from build123d import *

# Parameters (mm, degrees)
BOSS_EXTRUDE1_DEPTH = 4.125
SKETCH2_R           = 5
BOSS_EXTRUDE2_DEPTH = 0.5
SKETCH3_R           = 3.5
CUT_EXTRUDE1_DEPTH  = 9
SKETCH4_R           = 0.375
CUT_EXTRUDE2_DEPTH  = 0.5
CIRPATTERN1_COUNT   = 3
BOSS_EXTRUDE3_START = 6.5
BOSS_EXTRUDE3_DEPTH = 6.5
SKETCH7_R           = 3.5
BOSS_EXTRUDE4_DEPTH = 6.5
SKETCH8_R           = 3
CUT_EXTRUDE3_DEPTH  = 9
SKETCH6_R           = 0.75
CUT_EXTRUDE4_DEPTH  = 9


with BuildPart() as part:
    # Sketch1 → Boss-Extrude1 (new, symmetric)
    with BuildSketch(Plane.XY):
        Polygon((3, 0), (-3, 0), (-3, -0.45), (-2.5, -0.45), (-2.5, -0.9), (-3, -0.9), (-3, -1.35), (-2.5, -1.35), (-2.5, -1.8), (-3, -1.8), (-3, -2.25), (-2.5, -2.25), (-2.5, -2.7), (-3, -2.7), (-3, -3.15), (-2.5, -3.15), (-2.5, -3.6), (-3, -3.6), (-3, -4.05), (-2.5, -4.05), (-2.5, -4.5), (-3, -4.5), (-3, -4.95), (-2.5, -4.95), (-2.5, -5.4), (-3, -5.4), (-3, -5.85), (-2.5, -5.85), (-2.5, -6.3), (2.5, -6.3), (2.5, -5.85), (3, -5.85), (3, -5.4), (2.5, -5.4), (2.5, -4.95), (3, -4.95), (3, -4.5), (2.5, -4.5), (2.5, -4.05), (3, -4.05), (3, -3.6), (2.5, -3.6), (2.5, -3.15), (3, -3.15), (3, -2.7), (2.5, -2.7), (2.5, -2.25), (3, -2.25), (3, -1.8), (2.5, -1.8), (2.5, -1.35), (3, -1.35), (3, -0.9), (2.5, -0.9), (2.5, -0.45), (3, -0.45), align=None)
    extrude(amount=BOSS_EXTRUDE1_DEPTH, both=True)

    # Sketch2 → Boss-Extrude2 (add)
    with BuildSketch(Plane.XY.offset(4.125)):
        with Locations(Location((0, -6, 0), (0, 0, 126.869897646))):
            Circle(SKETCH2_R)
    extrude(amount=BOSS_EXTRUDE2_DEPTH)

    # Sketch3 → Cut-Extrude1 (cut)
    with BuildSketch(Plane.XY.offset(4.625)):
        with Locations((0, -6)):
            Circle(SKETCH3_R)
    extrude(amount=-CUT_EXTRUDE1_DEPTH, mode=Mode.SUBTRACT)

    # Sketch4 → Cut-Extrude2 (cut)
    with BuildSketch(Plane.XY.offset(4.625)):
        with Locations((3.464101615, -4)):
            Circle(SKETCH4_R)
    cut_extrude2 = extrude(amount=-CUT_EXTRUDE2_DEPTH, mode=Mode.SUBTRACT)

    # CirPattern1: Cut-Extrude2 ×3 about axis
    cirpattern1_axis = Axis((0, -6, 0), (0, 0, 1))
    for i in range(1, CIRPATTERN1_COUNT):
        add(cut_extrude2.rotate(cirpattern1_axis, i * 360 / CIRPATTERN1_COUNT), mode=Mode.SUBTRACT)

    # Sketch5 → Boss-Extrude3 (add)
    with BuildSketch(Plane.XY.offset(-4.875).offset(BOSS_EXTRUDE3_START)):
        with BuildLine():
            Line((6, -12.75), (-6, -12.75))
            Line((-6, -12.75), (-3.312648335, -4.870238517))
            ThreePointArc((-3.312648335, -4.870238517), (0, -2.5), (3.312648335, -4.870238517))
            Line((3.312648335, -4.870238517), (6, -12.75))
        make_face()
    extrude(amount=-BOSS_EXTRUDE3_DEPTH)

    # Sketch7 → Boss-Extrude4 (add)
    with BuildSketch(Plane.XY.offset(4.625)):
        with Locations(Location((0, -6, 0), (0, 0, 161.168324383))):
            Circle(SKETCH7_R)
    extrude(amount=-BOSS_EXTRUDE4_DEPTH)

    # Sketch8 → Cut-Extrude3 (cut)
    with BuildSketch(Plane.XY.offset(4.625)):
        with Locations((0, -6)):
            Circle(SKETCH8_R)
    extrude(amount=-CUT_EXTRUDE3_DEPTH, mode=Mode.SUBTRACT)

    # Sketch6 → Cut-Extrude4 (cut)
    with BuildSketch(Plane(origin=(0, 0, -4.875), x_dir=(-1, 0, 0), z_dir=(0, 0, -1))):
        with Locations((0, -6)):
            Circle(SKETCH6_R)
    extrude(amount=-CUT_EXTRUDE4_DEPTH, mode=Mode.SUBTRACT)


solid = part.part
Here's how the part is built. I have some questions about the finished solid (model axes, mm). A direction names the side the tool comes from. Round coordinates to 2 decimals unless told otherwise and drop trailing zeros. Order: outer loops, then holes, each group sorted by start corner. A loop starts at its lowest first (then second) coordinate and runs counter-clockwise, first axis right, second up. Notation, with made-up numbers: (-7.5, -37) -> (28.5, -37) arc R13 ccw to (28.5, -30) -> close; hole circle Ø9 at (-27.75, -20). An arc over 180 degrees is marked (long way). Return JSON: item names as keys, results as strings.
Q1. Which directions (+Z, -Z, +X, -X, +Y, -Y) give clear straight access to the entire face, cutting with the end or side of a thin tool? Please do faces 1 (the flat face through (4.638, -8.755, -1.58)), 2 (the flat face through (0, -0.6, 4.125)), 3 (the cylindrical face through (2.82, -10.13, 4.37)), 4 (the flat face through (-2, -3, 4.625)), 5 (the cylindrical face through (0.326, -9.485, 1.979)).
Filled sheet:
{"face 1": "-Z, +X, +Y", "face 2": "+Z, +Y", "face 3": "+Z", "face 4": "+Z, +X, -X, +Y, -Y", "face 5": "none"}
Q2. For pin 1 Ø3.5 at (x, y) = (0, -6) entering from +Z (3 decimals); pin 2 Ø4 at (y, z) = (-3.5, 3) entering from -X; pin 3 Ø4 at (y, z) = (-8, -3) entering from +X, each with a flat end and sliding along its axis, tell me the tip position at first contact or that it passes through.
Filled sheet:
{"pin 1": "stops at z = -4.375", "pin 2": "stops at x = -4.93", "pin 3": "stops at x = 5.06"}
Q3. If we section it at D-D on x = 2: List the corners of the cut face in (y, z) for me (3 decimals).
Filled sheet:
{"outline": "(-12.75, -4.875) -> (-3.128, -4.875) -> (-3.128, -4.125) -> (0, -4.125) -> (0, 4.125) -> (-1.417, 4.125) -> (-1.417, 4.625) -> (-3.764, 4.625) -> (-3.764, -4.375) -> (-8.236, -4.375) -> (-8.236, 4.625) -> (-10.583, 4.625) -> (-10.583, 4.125) -> (-8.872, 4.125) -> (-8.872, 1.625) -> (-12.75, 1.625) -> close"}
Q4. I need wall thicknesses on line 1 along Y through (x, z) = (0, -2.25); line 2 along Z through (x, y) = (0.5, -9.5) (3 decimals); line 3 along Z through (x, y) = (4.75, -5) (3 decimals). Which ranges of each line are inside material? Lowest first, please. Write a range as from..to.
Filled sheet:
{"line 1": "y = -12.75..-9, -3..0", "line 2": "z = -4.875..1.625, 4.125..4.625", "line 3": "z = 4.125..4.625"}
Q5. If we section it at C-C on y = -10: List the corners of the cut face in (x, z) for me (3 decimals).
Filled sheet:
{"outline": "(-5.062, -4.875) -> (5.062, -4.875) -> (5.062, 1.625) -> (-5.062, 1.625) -> close; (-3, 4.125) -> (-0.375, 4.125) -> (-0.375, 4.625) -> (-3, 4.625) -> close; (0.375, 4.125) -> (3, 4.125) -> (3, 4.625) -> (0.375, 4.625) -> close"}
Q6. If we mould it in two halves opening along X, with no side actions, what happens to faces 6 (the flat face through (1, -7, -4.375)), 7 (the flat face through (-4.675, -8.865, -1.58)), 8 (the cylindrical face through (0, -3, 0)), 9 (the flat face through (0, -1, -4.125))? For each: released by +X, released by -X, zero draft, split by the parting line, or undercut.
Filled sheet:
{"face 6": "undercut", "face 7": "released by -X", "face 8": "undercut", "face 9": "zero draft"}
Q7. If we section it at A-A on x = 0: List the corners of the cut face in (y, z) for me (3 decimals).
Filled sheet:
{"outline": "(-12.75, -4.875) -> (-6.75, -4.875) -> (-6.75, -4.375) -> (-9, -4.375) -> (-9, 4.625) -> (-9.625, 4.625) -> (-9.625, 4.125) -> (-9.5, 4.125) -> (-9.5, 1.625) -> (-12.75, 1.625) -> close; (-11, 4.125) -> (-10.375, 4.125) -> (-10.375, 4.625) -> (-11, 4.625) -> close; (-5.25, -4.875) -> (-2.5, -4.875) -> (-2.5, -4.125) -> (0, -4.125) -> (0, 4.125) -> (-1, 4.125) -> (-1, 4.625) -> (-3, 4.625) -> (-3, -4.375) -> (-5.25, -4.375) -> close"}
Q8. If we section it at B-B on y = -6.25: List the corners of the cut face in (x, z) for me (3 decimals), plus the area to 3 significant figures.
Filled sheet:
{"outline": "(-4.994, 4.125) -> (-3.491, 4.125) -> (-3.491, 1.625) -> (-3.783, 1.625) -> (-3.783, -4.875) -> (-0.707, -4.875) -> (-0.707, -4.375) -> (-2.99, -4.375) -> (-2.99, 4.625) -> (-4.994, 4.625) -> close; (0.707, -4.875) -> (3.783, -4.875) -> (3.783, 1.625) -> (3.491, 1.625) -> (3.491, 4.125) -> (4.994, 4.125) -> (4.994, 4.625) -> (2.99, 4.625) -> (2.99, -4.375) -> (0.707, -4.375) -> close", "area": "17.1 mm^2"}
